Autodesk Inventor part; units mm, degrees
ref_plane "Work Plane1" through (60, 0, 0) normal (1, 0, 0) x (0, 1, 0)
ref_plane "Work Plane2" through (60, 0, 0) normal (1, 0, 0) x (0, 1, 0)
ref_plane "XZ Plane" through (0, 0, 0) normal (0, 1, 0) x (-1, 0, 0)
sketch "Sketch1" plane through (0, 0, 0) normal (0, 0, 1) x (1, 0, 0)
  line L0 (0, 0) -> (0, 66)
  line L1 (75, -0.1929) -> (75, 14.8071)
  line L2 (-21.5975, 0) -> (0, 0)
  line L3 (46.9201, 0) -> (53.1744, 0)
  line L4 (75, 14.8071) -> (60, 14.8071)
  line L5 (60, 14.8071) -> (60, 34.8071)
  line L6 (0, 33.8071) -> (0, 49.8071)
  line L7 (0, 49.8071) -> (35, 49.8071)
  line L8 (46.9201, 9.8071) -> (40, 9.8071)
  line L9 (40, 9.8071) -> (40, 33.8071)
  line L10 (60, 34.8071) -> (60, 49.8071)
  line L11 (60, 49.8071) -> (35, 49.8071)
  line L12 (46.9201, 9.8071) -> (50, 9.8071)
  line L13 (50, 9.8071) -> (50, -0.1929)
  line L14 (50, -0.1929) -> (75, -0.1929)
  line L15 (0, 33.8071) -> (0, 9.8071)
  line L16 (0, 9.8071) -> (20, 9.8071)
  line L17 (20, 9.8071) -> (20, 33.8071)
  line L18 (20, 33.8071) -> (40, 33.8071)
  dimension "d0" = 66
  dimension "d2" = 150
  dimension "d4" = 15
  dimension "d5" = 20
  dimension "d15" = 35
  dimension "d16" = 70
  dimension "d84" = 100
  dimension "d92" = 50
  dimension "d132" = 15
  dimension "d134" = 10
  dimension "d136" = 40
  dimension "d137" = 20
revolve "Revolution1" add sketch "Sketch1" angle 360 about axis through (0, 0, 0) along (0, 1, 0)
chamfer "Chamfer1" distance 20 angle 45 1 edges at (-60, 49.8071, 0)
ref_plane "Work Plane1" through (60, 0, 0) normal (1, 0, 0) x (0, 1, 0)
sketch "Sketch10" plane through (0, 49.8071, 0) normal (0, 1, 0) x (1, 0, 0)
  circle A0 centre (0, 0) radius 16
  dimension "d54" = 32
hole "Hole2" at (0, 49.8071, 0) direction (0, -1, 0) diameter 35 end through all
ref_plane "Work Plane2" through (60, 0, 0) normal (1, 0, 0) x (0, 1, 0)
sketch "Sketch14" plane through (60, 0, 0) normal (1, 0, 0) x (0, 1, 0)
  circle A0 centre (45.5775, 0) radius 5
  point P0 (0, 0)
  dimension "d89" = 10
sketch "Sketch15" plane through (0, 0, 0) normal (0, 0, 1) x (1, 0, 0)
  line L0 (59.908, 45.3055) -> (36.1068, 21.3737)
  point P0 (0, 0)
sweep "Sweep4" cut profiles "Sketch14" path "Sketch15"
sketch "Sketch18" plane through (0, 49.8071, 0) normal (0, 1, 0) x (1, 0, 0)
  point P0 (0, 0)
sketch "Sketch19" plane through (0, 49.8071, 0) normal (0, 1, 0) x (1, 0, 0)
  circle A0 centre (-21, 0) radius 2
  circle A1 centre (-10.5, -18.1865) radius 2
  circle A2 centre (10.5, -18.1865) radius 2
  circle A3 centre (21, 0) radius 2
  circle A4 centre (10.5, 18.1865) radius 2
  circle A5 centre (-10.5, 18.1865) radius 2
  point P0 (0, 0)
  dimension "d144" = 4
  dimension "d145" = 21
  dimension "d148" = 360
hole "Hole5" at (-21, 49.8071, 0) at (-10.5, 49.8071, -18.1865) at (21, 49.8071, 0) at (10.5, 49.8071, 18.1865) at (-10.5, 49.8071, 18.1865) at (10.5, 49.8071, -18.1865) direction (0, -1, 0) diameter 4 depth 5 tip angle 118
thread "Thread21"
thread "Thread22"
thread "Thread23"
thread "Thread24"
thread "Thread25"
thread "Thread26"
equation "\"d60\" = Thickness"
equation "\"BendRadius\" = Thickness"
equation "\"BendReliefWidth\" = Thickness"
equation "\"BendReliefDepth\" = 0.5 * Thickness"
equation "\"CornerReliefSize\" = 4 * Thickness"
equation "\"MinimumRemnant\" = 2 * Thickness"
equation "\"TransitionRadius\" = BendRadius"
equation "\"JacobiRadiusSize\" = BendRadius"
equation "\"GapSize\" = Thickness"
properties material "Stainless Steel"
Work out the finished part from the listing and answer in its coordinate system (mm). A direction names the side the tool comes from. Coordinates: 2 decimals unless noted, no trailing zeros. Loops run counter-clockwise (first coordinate to the right, second up) from the corner with the lowest first, then second, coordinate; pieces in that order, holes last. Notation, with made-up numbers: M 8.5,65.5 L 15.5,65.5 A22 ccw 15.5,90.5 Z; hole C 51.25,77.25 d11. An arc over 180 degrees is marked long. Answer in a Markdown table with one row per item. Add a question column.
1. Flat-ended cylindrical pins translate along their axes: P1, Ø1.5, axis at x = -32, y = 12, coming from the +Z side; P2, Ø6, axis at y = 19.5, z = -5.5, coming from the -X side; P3, Ø1.5, axis at x = -13.5, y = 45, coming from the +Z side. Find the tip coordinate at first contact, or state that the pin passes through.
2. A tool of negligible diameter and unlimited length cuts with its end or side. For faces 1 (the cylindrical face through (8.814, 47.272, 19.262)), 2 (the cylindrical face through (10.648, 29.527, -13.887)), 3 (the cylindrical face through (-8.67, 21.98, 39.05)), from which of +Z, -Z, +X, -X, +Y, -Y can it reach the whole face along a straight path? Write none if from no direction.
3. The mould has two halves that part along Z. Classify faces 4 (the flat face through (-9.4, 33.807, -18.3)), 5 (the cylindrical face through (-13.007, 22.412, 58.573)), 6 (the flat face through (49, -0.193, 16)): pulls with the +Z half, pulls with the -Z half, needs draft (parallel to the pull), parting line crosses it, or undercut.
4. Consider L1, parallel to Z at x = 0, y = 4.5; L2, parallel to X at y = 21.5, z = 0; L3, parallel to Y at x = -44.5, z = -44. Determine where each line is inside the solid, lowest interval first.
5. Find section A-A, the plane y = 4. Write down the section's boundary in (x, z), then the cut area to 3 significant figures.
Reported:
| question | item | result |
|---|---|---|
| 1 | P1 | stops at z = 68.18 |
| 1 | P2 | stops at x = -59.95 |
| 1 | P3 | stops at z = 43.54 |
| 2 | face 1 | +Y |
| 2 | face 2 | +Y, -Y |
| 2 | face 3 | -Y |
| 3 | face 4 | undercut |
| 3 | face 5 | parting line crosses it |
| 3 | face 6 | needs draft |
| 4 | L1 | z = -75 to -50, 50 to 75 |
| 4 | L2 | x = -60 to -40, -20 to -17.5, 17.5 to 20, 41.03 to 60 |
| 4 | L3 | y = -0.19 to 14.81 |
| 5 | outline | C 0,0 d150; hole C 0,0 d100 |
| 5 | area | 9,820 mm^2 |
